Design review of the part built by this model. Coordinates are the model's own, in mm. A direction names the side the tool comes from. Coordinates: 2 decimals unless noted, no trailing zeros. Loops run counter-clockwise (first coordinate to the right, second up) from the corner with the lowest first, then second, coordinate; pieces in that order, holes last.
Q1. Wall thickness on probe 1 along X at (y, z) = (-0.25, 5) (3 decimals); probe 2 along Y at (x, z) = (3.75, 5.25); probe 3 along Z at (x, y) = (5.5, -1.75) (3 decimals): over which ranges is each line inside the solid? List them lowest first.
Q2. Add section B-B on z = -2.5. Give the boundary of the cut face in (x, y) (3 decimals).
Q3. Machinability: for faces 1 (the face through (6, -1, -7.825)), 2 (the face through (6.465, -1, 0)), 3 (the face through (-4.865, -1, 0)), which of the approach directions +Z, -Z, +X, -X, +Y, -Y give a long, thin tool a straight path to every point of the face, cutting with its end or side? Answer none if there is none.
Q4. Add section C-C on x = 1.75. Give the boundary of the cut face in (y, z) (3 decimals), and give its area (3 significant figures).
Q5. Add section A-A on y = -0.5. Give the boundary of the cut face in (x, z) (3 decimals), and give its area (3 significant figures).
Q6. For P1, Ø1, axis at y = -1.5, z = 1, coming from the +X side (3 decimals); P2, Ø0.8, axis at x = -5.5, y = -1, coming from the -Z side (3 decimals); P3, Ø0.8, axis at x = 6, y = -1, coming from the +Z side (3 decimals), all flat-tipped, find the tip position at first contact; note any pin that passes through.
Q7. Draft analysis for pull direction X (two halves, no side actions). For faces 4 (the face through (0, 0, 0)), 5 (the face through (-6, -1, 7.825)), 6 (the face through (-6.465, -1, 0)), state which applies: released by +X, released by -X, zero draft, split by the parting line, or undercut.
Autodesk Inventor part; units mm, degrees
ref_plane "YZ Plane" through (0, 0, 0) normal (1, 0, 0) x (0, 1, 0)
ref_plane "XZ Plane" through (0, 0, 0) normal (0, 1, 0) x (-1, 0, 0)
ref_plane "XY Plane" through (0, 0, 0) normal (0, 0, 1) x (1, 0, 0)
sketch "Sketch1" plane through (0, 0, 0) normal (0, 1, 0) x (-1, 0, 0)
  line L0 (-6.665, 8.025) -> (6.665, 8.025)
  line L1 (6.665, 8.025) -> (6.665, -8.025)
  line L2 (6.665, -8.025) -> (-6.665, -8.025)
  line L3 (-6.665, -8.025) -> (-6.665, 8.025)
  line L4 (-6.665, 8.025) -> (6.665, -8.025) construction
  line L5 (6.665, 8.025) -> (-6.665, -8.025) construction
  line L6 (0, -11.235) -> (0, 11.235)
  line L7 (6.665, 8.025) -> (4.665, 8.025)
  line L8 (4.665, 8.025) -> (4.665, -8.025)
  line L9 (4.665, -8.025) -> (6.665, -8.025)
  line L10 (6.665, -8.025) -> (6.665, 8.025)
  line L11 (-6.665, -8.025) -> (-4.665, -8.025)
  line L12 (-4.665, -8.025) -> (-4.665, 8.025)
  line L13 (-4.665, 8.025) -> (-6.665, 8.025)
  line L14 (-6.665, 8.025) -> (-6.665, -8.025)
  line L15 (4.865, -7.825) -> (4.865, 7.825)
  line L16 (4.865, 7.825) -> (6.465, 7.825)
  line L17 (6.465, 7.825) -> (6.465, -7.825)
  line L18 (6.465, -7.825) -> (4.865, -7.825)
  line L19 (-6.465, -7.825) -> (-4.865, -7.825)
  line L20 (-4.865, -7.825) -> (-4.865, 7.825)
  line L21 (-4.865, 7.825) -> (-6.465, 7.825)
  line L22 (-6.465, 7.825) -> (-6.465, -7.825)
  point P0 (0, 0)
  dimension "d0" = 16.05
  dimension "d1" = 13.33
  dimension "d7" = 2
  dimension "d8" = 0.2
  dimension "d9" = 0.2
extrude "Extrusion1" add sketch "Sketch1" along normal blind 2 contours L0 L12 L2 L3 | L0 L6 L2 L12 | L0 L8 L2 L6 | L0 L1 L2 L8 | L15 L16 L17 L18 | L22 L21 L20 L19
extrude "Extrusion2" add sketch "Sketch1" against normal blind 2 contours L15 L16 L17 L18 | L22 L21 L20 L19
chamfer "Chamfer1" distance 0.3 angle 45 8 edges at (-4.865, -1, 7.825) (-6.465, -1, 7.825) (4.865, -1, 7.825) (6.465, -1, 7.825) (4.865, -1, -7.825) (6.465, -1, -7.825) (-4.865, -1, -7.825) (-6.465, -1, -7.825)
properties part number "Logic_Level_Shifter"
Entries:
1. probe 1: x = -6.465 to -4.865, 4.865 to 6.465
1. probe 2: y = 0 to 2
1. probe 3: z = -7.825 to 7.825
2. outline: (-6.665, 0) - (-6.465, 0) - (-6.465, -2) - (-4.865, -2) - (-4.865, 0) - (4.865, 0) - (4.865, -2) - (6.465, -2) - (6.465, 0) - (6.665, 0) - (6.665, 2) - (-6.665, 2) - close
3. face 1: -Z, +X, -X, -Y
3. face 2: +Z, -Z, +X, -Y
3. face 3: +Z, -Z, -Y
4. outline: (0, -8.025) - (2, -8.025) - (2, 8.025) - (0, 8.025) - close
4. area: 32.1 mm2
5. outline: (-6.465, -7.525) - (-6.165, -7.825) - (-5.165, -7.825) - (-4.865, -7.525) - (-4.865, 7.525) - (-5.165, 7.825) - (-6.165, 7.825) - (-6.465, 7.525) - close; (4.865, -7.525) - (5.165, -7.825) - (6.165, -7.825) - (6.465, -7.525) - (6.465, 7.525) - (6.165, 7.825) - (5.165, 7.825) - (4.865, 7.525) - close
5. area: 49.7 mm2
6. P1: stops at x = 6.465
6. P2: stops at z = -7.825
6. P3: stops at z = 7.825
7. face 4: undercut
7. face 5: zero draft
7. face 6: released by -X
